```python
from build123d import *

# Parameters (mm, degrees)
SKETCH1_R           = 10.025
BOSS_EXTRUDE1_DEPTH = 2.2
SKETCH2_R           = 0.5
CUT_EXTRUDE1_DEPTH  = 3.2
SKETCH3_R           = 3.8
BOSS_EXTRUDE2_DEPTH = 3.4
SKETCH4_R           = 3
CUT_EXTRUDE2_DEPTH  = 2.8
SKETCH5_R           = 1.25
CUT_EXTRUDE3_DEPTH  = 3.8


with BuildPart() as part:
    # Sketch1 → Boss-Extrude1 (new body)
    with BuildSketch(Plane(origin=(0, 0, 0), x_dir=(1, 0, 0), z_dir=(0, 1, 0))):
        Circle(SKETCH1_R)
    extrude(amount=BOSS_EXTRUDE1_DEPTH)

    # Sketch2 → Cut-Extrude1 (cut, through all)
    with BuildSketch(Plane.XZ):
        with Locations((-7.025, -3)):
            Circle(SKETCH2_R)
        with Locations((-7.025, 0)):
            Circle(SKETCH2_R)
        with Locations((-7.025, 3)):
            Circle(SKETCH2_R)
        with Locations((-3, 7.025)):
            Circle(SKETCH2_R)
        with Locations((0, 7.025)):
            Circle(SKETCH2_R)
        with Locations((3, 7.025)):
            Circle(SKETCH2_R)
        with Locations((7.025, 3)):
            Circle(SKETCH2_R)
        with Locations((7.025, 0)):
            Circle(SKETCH2_R)
        with Locations((7.025, -3)):
            Circle(SKETCH2_R)
        with Locations((3, -7.025)):
            Circle(SKETCH2_R)
        with Locations((0, -7.025)):
            Circle(SKETCH2_R)
        with Locations((-3, -7.025)):
            Circle(SKETCH2_R)
    extrude(amount=-CUT_EXTRUDE1_DEPTH, mode=Mode.SUBTRACT)

    # Sketch3 → Boss-Extrude2 (add)
    with BuildSketch(Plane(origin=(0, 0, 0), x_dir=(-1, 0, 0), z_dir=(0, -1, 0))):
        Circle(SKETCH3_R)
    extrude(amount=BOSS_EXTRUDE2_DEPTH)

    # Sketch4 → Cut-Extrude2 (cut)
    with BuildSketch(Plane.XZ.offset(3.4)):
        Circle(SKETCH4_R)
    extrude(amount=-CUT_EXTRUDE2_DEPTH, mode=Mode.SUBTRACT)

    # Sketch5 → Cut-Extrude3 (cut, through all)
    with BuildSketch(Plane.XZ.offset(0.6)):
        Circle(SKETCH5_R)
    extrude(amount=-CUT_EXTRUDE3_DEPTH, mode=Mode.SUBTRACT)


solid = part.part
```
Build history of the part. All positions in model axes, mm. A direction names the side the tool comes from. Round coordinates to 2 decimals unless told otherwise and drop trailing zeros. Loops run counter-clockwise (first coordinate to the right, second up) from the corner with the lowest first, then second, coordinate; pieces in that order, holes last. Notation, with made-up numbers: M -36,6 L 15,6 A19 ccw 15,35 Z; hole C 28,79 d10. An arc over 180 degrees is marked long. Answer as CSV lines item,"result".
1. Cut at A-A on z = 0. Write the cut outline in (x, y) (3 decimals).
Resolved:
outline,"M -10.025,0 L -7.525,0 L -7.525,2.2 L -10.025,2.2 Z; M -6.525,0 L -3.8,0 L -3.8,-3.4 L -3,-3.4 L -3,-0.6 L -1.25,-0.6 L -1.25,2.2 L -6.525,2.2 Z; M 1.25,-0.6 L 3,-0.6 L 3,-3.4 L 3.8,-3.4 L 3.8,0 L 6.525,0 L 6.525,2.2 L 1.25,2.2 Z; M 7.525,0 L 10.025,0 L 10.025,2.2 L 7.525,2.2 Z"
2. Wall check: probe 1 along Z at (x, y) = (0, 0.65) (3 decimals); probe 2 along Z at (x, y) = (3, 0.5) (3 decimals); probe 3 along Z at (x, y) = (0, -1.45). Give the ranges that are in metal, low to high. Write a range as [from, to].
Resolved:
probe 1,"z = [-10.025, -7.525], [-6.525, -1.25], [1.25, 6.525], [7.525, 10.025]"
probe 2,"z = [-9.566, -7.525], [-6.525, 6.525], [7.525, 9.566]"
probe 3,"z = [-3.8, -3], [3, 3.8]"
3. Two-plate mould, pull along X, no slides. Class faces 1 (the flat face through (2, 2.2, 0)), 2 (the cylindrical face through (-7.955, 1.085, 6.1)), 3 (the cylindrical face through (-3.07, 1.08, 7.52)): released by +X, released by -X, zero draft, split by the parting line, or undercut.
Resolved:
face 1,"zero draft"
face 2,"split by the parting line"
face 3,"undercut"
4. 3-axis set-ups, long thin cutter, end or side, ignore diameter. For faces 4 (the cylindrical face through (2.93, 1.08, 7.52)), 5 (the cylindrical face through (-3, -2, 0)): which of +Z, -Z, +X, -X, +Y, -Y reach the whole face in a straight line?
Resolved:
face 4,"+Y, -Y"
face 5,"-Y"
5. Flat gauge pins, fed straight in: P1, Ø1.5, axis at y = -2, z = -7, coming from the -X side; P2, Ø1, axis at y = 1, z = -7.5, coming from the -X side; P3, Ø1.8, axis at x = 0.5, z = 1, coming from the -Y side; P4, Ø1, axis at y = -1.5, z = -3.5, coming from the -X side. Where does each tip first touch, or does it go through?
Resolved:
P1,"passes through"
P2,"stops at x = -7.18"
P3,"stops at y = -0.6"
P4,"stops at x = -2.33"
6. Cut at B-B on x = 0. Write the cut outline in (y, z) (3 decimals), then the cut area to 4 significant figures.
Resolved:
outline,"M -3.4,-3.8 L 0,-3.8 L 0,-6.525 L 2.2,-6.525 L 2.2,-1.25 L -0.6,-1.25 L -0.6,-3 L -3.4,-3 Z; M -3.4,3 L -0.6,3 L -0.6,1.25 L 2.2,1.25 L 2.2,6.525 L 0,6.525 L 0,3.8 L -3.4,3.8 Z; M 0,-10.025 L 2.2,-10.025 L 2.2,-7.525 L 0,-7.525 Z; M 0,7.525 L 2.2,7.525 L 2.2,10.025 L 0,10.025 Z"
area,"41.75 mm²"
7. Cut at C-C on y = -2.25. Write the cut outline in (x, z), then the cut area to 3 significant figures.
Resolved:
outline,"C 0,0 d7.6; hole C 0,0 d6"
area,"17.1 mm²"
8. Cut at D-D on x = 3.25. Write the cut outline in (y, z).
Resolved:
outline,"M -3.4,-1.97 L 0,-1.97 L 0,-6.59 L 2.2,-6.59 L 2.2,6.59 L 0,6.59 L 0,1.97 L -3.4,1.97 Z; M 0,-9.48 L 2.2,-9.48 L 2.2,-7.46 L 0,-7.46 Z; M 0,7.46 L 2.2,7.46 L 2.2,9.48 L 0,9.48 Z"
